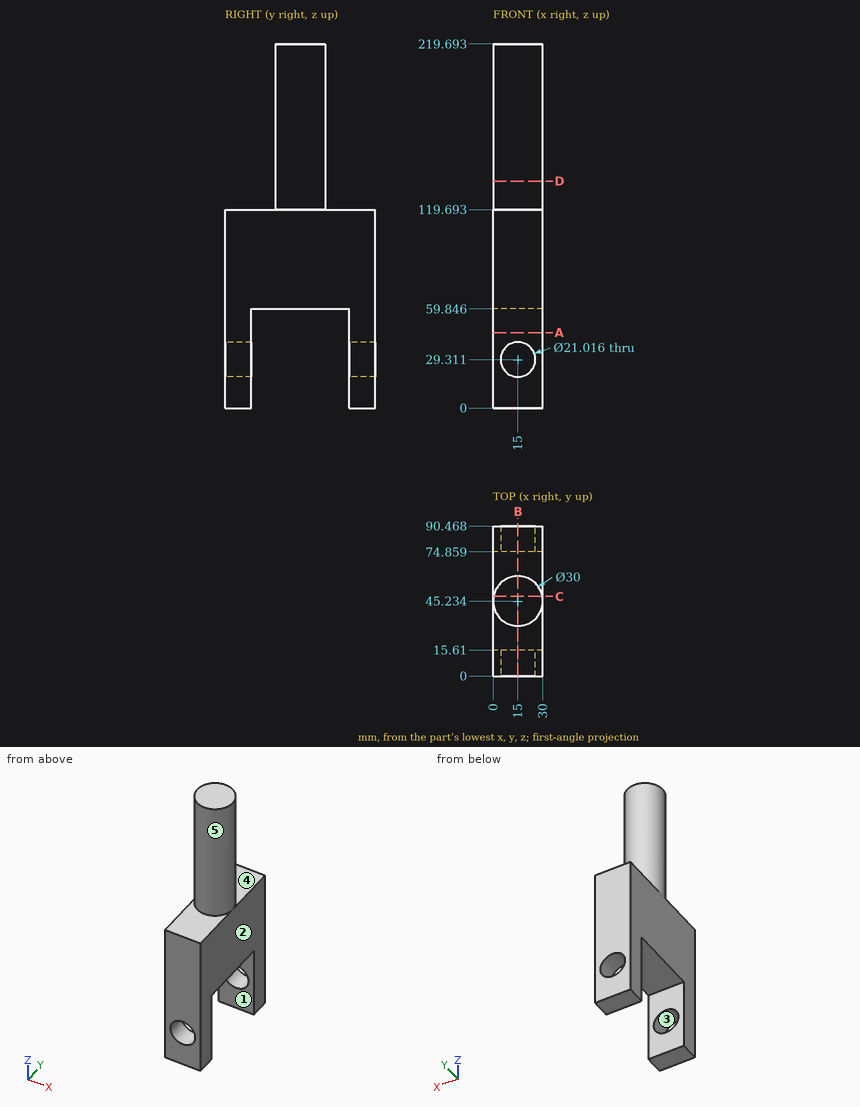
Job drawing, mm, ordinate dimensions from the low corner. One solid piece. A direction names the side the tool comes from. Coordinates: 2 decimals unless noted, no trailing zeros. Loops run counter-clockwise (first coordinate to the right, second up) from the corner with the lowest first, then second, coordinate; pieces in that order, holes last. Notation, with made-up numbers: (-37, 26.25) - (-19, 26.25) arc R21 cw to (-19, 47.25) - close; hole circle Ø4 at (-30, 33). An arc over 180 degrees is marked (long way). Write item = value, one per line. Start each with the question number.
Q1. Drill centre lines: L1, parallel to Z at x = 15, y = 81.25; L2, parallel to Y at x = 4, z = 37; L3, parallel to Z at x = 26.5, y = 15. Where is each one in solid material? Low to high.
Q2. Pull direction X, two halves, no side cores. Call the marked faces 3, 4 and 5: pulls with the +X half, pulls with the -X half, needs draft (parallel to the pull), parting line crosses it, or undercut.
Q3. Cut at C-C, the plane y = 48. List the corners of the cut face in (x, z).
Q4. Cut at B-B, the plane x = 15. List the corners of the cut face in (y, z) (1 decimal).
Q5. Which spindle directions (+Z, -Z, +X, -X, +Y, -Y) get a long thin tool onto all of the face, cutting with end or side? Do the marked faces 1 and 2. Say none if no direction does.
Q6. Cut at A-A, the plane z = 45.5. List the corners of the cut face in (x, y).
Q7. Flat gauge pins, fed straight in: pin 1 Ø1 at (x, z) = (23, 165.5) entering from +Y (1 decimal); pin 2 Ø5 at (x, z) = (13, 168.5) entering from +Y; pin 3 Ø5 at (x, y) = (7.5, 24) entering from -Z. Where does each tip first touch, or does it go through?
Q8. Cut at D-D, the plane z = 137. List the corners of the cut face in (x, y) (1 decimal).
Computed:
q1.L1 = 0 to 18.8, 39.82 to 119.69
q1.L2 = 0 to 15.61, 74.86 to 90.47
q1.L3 = 0 to 119.69
q2.face_3 = undercut
q2.face_4 = needs draft
q2.face_5 = parting line crosses it
q3.outline = (0, 59.85) - (30, 59.85) - (30, 119.69) - (29.74, 119.69) - (29.74, 219.69) - (0.26, 219.69) - (0.26, 119.69) - (0, 119.69) - close
q4.outline = (0, 0) - (15.6, 0) - (15.6, 18.8) - (0, 18.8) - close; (0, 39.8) - (15.6, 39.8) - (15.6, 59.8) - (74.9, 59.8) - (74.9, 39.8) - (90.5, 39.8) - (90.5, 119.7) - (60.2, 119.7) - (60.2, 219.7) - (30.2, 219.7) - (30.2, 119.7) - (0, 119.7) - close; (74.9, 0) - (90.5, 0) - (90.5, 18.8) - (74.9, 18.8) - close
q5.face_1 = -Z, +X, -X
q5.face_2 = +Z, -Z, +X, +Y, -Y
q6.outline = (0, 0) - (30, 0) - (30, 15.61) - (0, 15.61) - close; (0, 74.86) - (30, 74.86) - (30, 90.47) - (0, 90.47) - close
q7.pin_1 = 58.2
q7.pin_2 = 60.23
q7.pin_3 = 59.85
q8.outline = circle Ø30 at (15, 45.2)
